Read the model definition and answer for the solid it produces. Units are mm, in the model's axes. Face numbers are marked on the shaded views. Coordinates: 2 decimals unless noted, no trailing zeros. Write each loop counter-clockwise with the first axis right and the second up, starting at its lowest first coordinate (ties: lowest second). Pieces come first, ordered by that corner, then holes.
from build123d import *

# Parameters (mm, degrees)
F0_R           = 50.8
F1_DEPTH       = 38.1
F3_D           = 6.35
F4_D           = 9.525
F4_CBORE_D     = 19.05
F4_CBORE_DEPTH = 6.35
F5_D           = 9.525
F5_CSINK_D     = 19.05
F5_CSINK_ANGLE = 82
F6_D           = 6.35
F7_D           = 13.4874


with BuildPart() as f1:
    # F0 (on Front) → F1 (new body)
    with BuildSketch(Plane.XZ):
        Circle(F0_R)
        with BuildLine():
            ThreePointArc((0, 31.75), (22.45064, 22.45064), (31.75, 0))
            ThreePointArc((31.75, 0), (-22.45064, -22.45064), (0, 31.75))
        make_face(mode=Mode.SUBTRACT)
        with BuildLine():
            ThreePointArc((0, 31.75), (-22.45064, -22.45064), (31.75, 0))
            ThreePointArc((31.75, 0), (22.45064, 22.45064), (0, 31.75))
        make_face()
    extrude(amount=F1_DEPTH)

    # F3 (through all)
    with Locations(Plane.XZ.offset(38.1)):
        with Locations((0, 31.75)):
            Hole(F3_D / 2)

    # F4 (through all)
    with Locations(Plane.XZ.offset(38.1)):
        with Locations((28.636823, 13.711123)):
            CounterBoreHole(F4_D / 2, F4_CBORE_D / 2, F4_CBORE_DEPTH)

    # F5 (through all)
    with Locations(Plane.XZ.offset(38.1)):
        with Locations((19.574312, -24.712568)):
            CounterSinkHole(F5_D / 2, F5_CSINK_D / 2, counter_sink_angle=F5_CSINK_ANGLE)

    # F6 (through all)
    with Locations(Plane.XZ.offset(38.1)):
        with Locations((-19.574312, -24.712568)):
            Hole(F6_D / 2)

    # F7 (through all)
    with Locations(Plane.XZ.offset(38.1)):
        with Locations((-28.636823, 13.711123)):
            Hole(F7_D / 2)


solid = f1.part
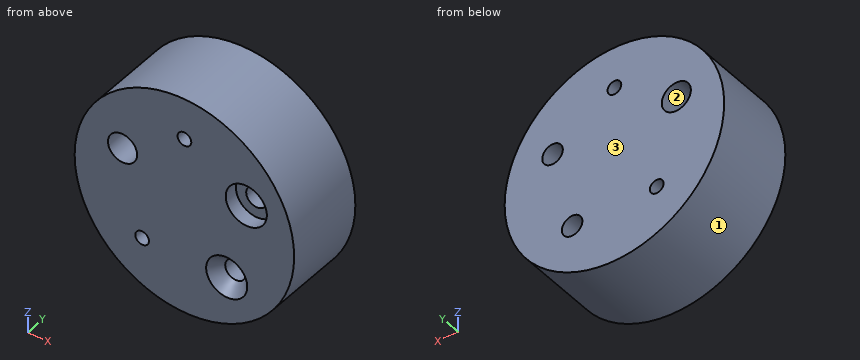
Item 1: The part is cut by section A-A (x = 0). Give the vertices of the cut face in (y, z) (3 decimals), and give its area (3 significant figures).
Item 2: The part is cut by section D-D (z = 12). Give the vertices of the cut face in (x, y), and give its area (3 significant figures).
Item 3: The part is cut by section B-B (z = 31.75). Give the vertices of the cut face in (x, y) (3 decimals), and give its area (3 significant figures).
Item 4: Given pin 1 (1 mm diameter, centred on x = 30.5, y = -21, fed in from -Z); pin 2 (2 mm diameter, centred on x = 19, y = -10.5, fed in from -Z); pin 3 (8 mm diameter, centred on y = -15.5, z = -29.5, fed in from +X), each flat-ended and moving along its own axis, determine where each tip first touches the part or whether it passes through.
Item 5: Determine the mould class of the marked faces 1, 2 and 3 for opening direction Z: +Z half, -Z half, draft (parallel to the pull), parting line (faces both ways), or undercut.
Item 6: Find the intervals of material crossed by probe 1 along X at (y, z) = (-8.5, 11); probe 2 along Z at (x, y) = (18, -30); probe 3 along X at (y, z) = (-6, 17.5), in increasing order.
Item 7: The part is cut by section C-C (y = -21.5). State how many separate pieces and enclosed holes the cut face has, and give its area (3 significant figures).
Answer:
1. outline: (-38.1, -50.8) - (0, -50.8) - (0, 28.575) - (-38.1, 28.575) - close; (-38.1, 34.925) - (0, 34.925) - (0, 50.8) - (-38.1, 50.8) - close
1. area: 3,630 mm2
2. outline: (-49.36, -38.1) - (-35.16, -38.1) - (-35.16, 0) - (-49.36, 0) - close; (-22.11, -38.1) - (19.27, -38.1) - (19.27, -31.75) - (24.19, -31.75) - (24.19, 0) - (-22.11, 0) - close; (33.08, -31.75) - (38.01, -31.75) - (38.01, -38.1) - (49.36, -38.1) - (49.36, 0) - (33.08, 0) - close
2. area: 2,860 mm2
3. outline: (-39.656, -38.1) - (-3.175, -38.1) - (-3.175, 0) - (-39.656, 0) - close; (3.175, -38.1) - (39.656, -38.1) - (39.656, 0) - (3.175, 0) - close
3. area: 2,780 mm2
4. pin 1: stops at z = -41
4. pin 2: stops at z = -47.5
4. pin 3: stops at x = 43.94
5. face 1: parting line
5. face 2: undercut
5. face 3: draft
6. probe 1: x = -49.59 to -34.81, -22.46 to 24.72, 32.55 to 49.59
6. probe 2: z = -47.5 to -29.21, -20.22 to 47.5
6. probe 3: x = -47.69 to -34.22, -23.06 to 25.75, 31.52 to 47.69
7. separate pieces: 1
7. enclosed holes: 5
7. area: 7,760 mm2
